Part model, mm, in its own coordinate system. Coordinates: 2 decimals unless noted, no trailing zeros. One line per question, with ' | ' between items. Start each with the question number.
from build123d import *

# Parameters (mm, degrees)
PAD012_DEPTH                = 3
CYLINDER047_R               = 1.75
CYLINDER047_DEPTH           = 18
CYLINDER047_ROLL_ANGLE      = -89.999776
CYLINDER047_PITCH_ANGLE     = 1.4e-05
CYLINDER047_PLACEMENT_ANGLE = -9.999925
CYLINDER042_R               = 3
CYLINDER042_DEPTH           = 3
CYLINDER042_ROLL_ANGLE      = -89.999776
CYLINDER042_PITCH_ANGLE     = 1.4e-05
CYLINDER042_PLACEMENT_ANGLE = -9.999925


with BuildPart() as obj1:
    # Sketch012 → Pad012 (new body)
    with BuildSketch(Plane.XY):
        with BuildLine():
            add(Edge.make_bspline(
                [(44.997663, -28.408983), (45.245046, -6.764399), (28.5, -0.316434)],
                knots=[1.556693, 1.556693, 1.556693, 2.83913, 2.83913, 2.83913], degree=2, weights=[1, 0.801368, 1]))
            Line((28.5, -0.316434), (28.5, -25.5))
            Line((28.5, -25.5), (44.997663, -28.408983))
        make_face()
    extrude(amount=PAD012_DEPTH)


with BuildPart() as obj1_1:
    # Body014 placement: moved
    add(obj1.part.moved(Location((0, 0, 2))))


with BuildPart() as cylinder047:
    # Cylinder047 → Cylinder047 (new body)
    with BuildSketch(Plane.XY):
        Circle(CYLINDER047_R)
    extrude(amount=CYLINDER047_DEPTH)


with BuildPart() as cylinder047_1:
    # Cylinder047 roll: moved
    add(cylinder047.part.rotate(Axis((0, 0, 0), (1, 0, 0)), CYLINDER047_ROLL_ANGLE))


with BuildPart() as cylinder047_2:
    # Cylinder047 pitch: moved
    add(cylinder047_1.part.rotate(Axis((0, 0, 0), (0, 1, 0)), CYLINDER047_PITCH_ANGLE))


with BuildPart() as cylinder047_3:
    # Cylinder047 placement: moved
    add(cylinder047_2.part.moved(Location((32.055183, -23.766017, 7.500006))).rotate(Axis((32.055183, -23.766017, 7.500006), (0, 0, 1)), CYLINDER047_PLACEMENT_ANGLE))


with BuildPart() as cut058:
    # Cylinder042 → Cylinder042 (new body)
    with BuildSketch(Plane.XY):
        Circle(CYLINDER042_R)
    extrude(amount=CYLINDER042_DEPTH)


with BuildPart() as cut058_1:
    # Cylinder042 roll: moved
    add(cut058.part.rotate(Axis((0, 0, 0), (1, 0, 0)), CYLINDER042_ROLL_ANGLE))


with BuildPart() as cut058_2:
    # Cylinder042 pitch: moved
    add(cut058_1.part.rotate(Axis((0, 0, 0), (0, 1, 0)), CYLINDER042_PITCH_ANGLE))


with BuildPart() as cut058_3:
    # Cylinder042 placement: moved
    add(cut058_2.part.moved(Location((34.141828, -11.94807, 7.500056))).rotate(Axis((34.141828, -11.94807, 7.500056), (0, 0, 1)), CYLINDER042_PLACEMENT_ANGLE))

    # Cut038: cut Cylinder047
    add(cylinder047_3.part, mode=Mode.SUBTRACT)

    # Cut058: cut obj1
    add(obj1_1.part, mode=Mode.SUBTRACT)


solid = cut058_3.part
1) Mould opens along X. For faces 1 (the flat face through (34, -10, 5)), 2 (the cylindrical face through (34.3, -10.5, 10.5)), 3 (the cylindrical face through (35.99, -10.77, 8.17)) say: +X half, -X half, draft (parallel to the pull), parting line (faces both ways), or undercut.
2) Pin check, flat tip, straight feed: pin 1 Ø1.5 at (x, z) = (32, 10) entering from -Y. Stop position of the tip, or through.
3) Wall check: line 1 along Z through (x, y) = (34, -10.1); line 2 along Z through (x, y) = (35.25, -12); line 3 along X through (y, z) = (-11.4, 6.45). Give the ranges that are in metal, low to high. Write a range as [from, to].
Values found:
1) face 1: draft | face 2: parting line | face 3: undercut
2) pin 1: y = -11.7
3) line 1: [5, 5.81], [9.19, 10.46] | line 2: [5, 6.14], [8.86, 10.29] | line 3: [31.38, 32.81], [35.66, 37.09]
